from build123d import *

# Parameters (mm, degrees)
SKIZZE1_W                       = 16
SKIZZE1_H                       = 8
SKIZZE1_R                       = 1.5
AUFSATZ_LINEAR_AUSTRAGEN1_DEPTH = 4.7
VERRUNDUNG1_R                   = 1
FASE1_SIZE                      = 1.5
SKIZZE2_R                       = 1.5
AUFSATZ_LINEAR_AUSTRAGEN2_DEPTH = 10


with BuildPart() as part:
    # Skizze1 → Aufsatz-Linear austragen1 (new body)
    with BuildSketch(Plane.XY):
        with Locations((-8, 0)):
            Rectangle(SKIZZE1_W, SKIZZE1_H)
        with Locations((-4, 0)):
            Circle(SKIZZE1_R, mode=Mode.SUBTRACT)
    extrude(amount=AUFSATZ_LINEAR_AUSTRAGEN1_DEPTH)

    # Verrundung1
    verrundung1_edges = [part.edges().sort_by_distance(p)[0] for p in [
        (0, -4, 2.35),
        (-16, -4, 2.35),
        (-16, 4, 2.35),
        (0, 4, 2.35),
    ]]
    fillet(verrundung1_edges, radius=VERRUNDUNG1_R)

    # Fase1
    fase1_edges = [part.edges().sort_by_distance(p)[0] for p in [
        (-5.5, 0, 4.7),
    ]]
    chamfer(fase1_edges, length=FASE1_SIZE)

    # Skizze2 → Aufsatz-Linear austragen2 (add)
    with BuildSketch(Plane(origin=(0, 0, 0), x_dir=(0, 0, -1), z_dir=(1, 0, 0))):
        with Locations((-2.25, 0)):
            Circle(SKIZZE2_R)
    extrude(amount=AUFSATZ_LINEAR_AUSTRAGEN2_DEPTH)


solid = part.part
Could you check a few things on this model? Use its own coordinates, in mm. A direction names the side the tool comes from. Give positions to 0.01 mm unless a question says otherwise; leave off trailing zeros. Order: outer loops, then holes, each group sorted by start corner. A loop starts at its lowest first (then second) coordinate and runs counter-clockwise, first axis right, second up. Notation, with made-up numbers: (-35, 13.5) - (12, 13.5) arc R7 ccw to (12, 17.5) - close; hole circle Ø7 at (80.25, 16). An arc over 180 degrees is marked (long way). One line per question, with ' | ' between items. Start each with the question number.
Item 1: Thinking about a two-plate mould opening in X: for faces 3 (the cylindrical face through (-2.614, -0.575, 1.578)), 4 (the flat face through (-8, -4, 2)), 5 (the flat face through (0, 0, 4)), 6 (the flat face through (-16, 0, 2)), which applies, pulls with the +X half, pulls with the -X half, needs draft (parallel to the pull), parting line crosses it, or undercut?
Item 2: I want a section at B-B on x = -4. Write out the boundary of the cut face in (y, z).
Item 3: I need wall thicknesses on probe 1 along Y at (x, z) = (-4, 2.35); probe 2 along X at (y, z) = (-1.75, 2.55); probe 3 along X at (y, z) = (0.5, 0.5). Which ranges of each line are inside material? Lowest first, please. Write a range as [from, to].
Item 4: I want a section at D-D on x = 0.5. Write out the boundary of the cut face in (y, z).
Item 5: I want a section at A-A on y = 0. Write out the boundary of the cut face in (x, z), then the cut area to 4 significant figures.
Item 6: I want a section at C-C on z = 2.25. Write out the boundary of the cut face in (x, y), then the cut area to 3 significant figures.
Item 7: I'm going to push flat-ended pins straight in: pin 1 Ø2.5 at (y, z) = (-1.5, 2.5) entering from +X; pin 2 Ø1.5 at (y, z) = (-2.5, 3.5) entering from +X; pin 3 Ø3 at (x, y) = (2.5, 1) entering from -Z. Where does each tip first touch, or does it pass through?
Item 8: For faces 1 (the cylindrical face through (4.93, 0.45, 0.82)), 2 (the cylindrical face through (-0.301, 3.715, 2.383)), which set-ups out of +Z, -Z, +X, -X, +Y, -Y let a thin tool reach every point of the face, with its end or its side?
Verdict:
1) face 3: undercut | face 4: needs draft | face 5: pulls with the +X half | face 6: pulls with the -X half
2) outline: (-4, 0) - (-1.5, 0) - (-1.5, 3.2) - (-3, 4.7) - (-4, 4.7) - close; (1.5, 0) - (4, 0) - (4, 4.7) - (3, 4.7) - (1.5, 3.2) - close
3) probe 1: [-4, -1.5], [1.5, 4] | probe 2: [-16, 0] | probe 3: [-16, -5.41], [-2.59, 0]
4) outline: circle Ø3 at (0, 2.25)
5) outline: (-16, 0) - (-5.5, 0) - (-5.5, 3.2) - (-7, 4.7) - (-16, 4.7) - close; (-2.5, 0) - (0, 0) - (0, 0.75) - (10, 0.75) - (10, 3.75) - (0, 3.75) - (0, 4.7) - (-1, 4.7) - (-2.5, 3.2) - close | area: 88.85 mm^2
6) outline: (-16, -3) arc R1 ccw to (-15, -4) - (-1, -4) arc R1 ccw to (0, -3) - (0, -1.5) - (10, -1.5) - (10, 1.5) - (0, 1.5) - (0, 3) arc R1 ccw to (-1, 4) - (-15, 4) arc R1 ccw to (-16, 3) - close; hole circle Ø3 at (-4, 0) | area: 150 mm^2
7) pin 1: x = 10 | pin 2: x = 0 | pin 3: z = 0.75
8) face 1: +X | face 2: +Z, -Z, +X, +Y
